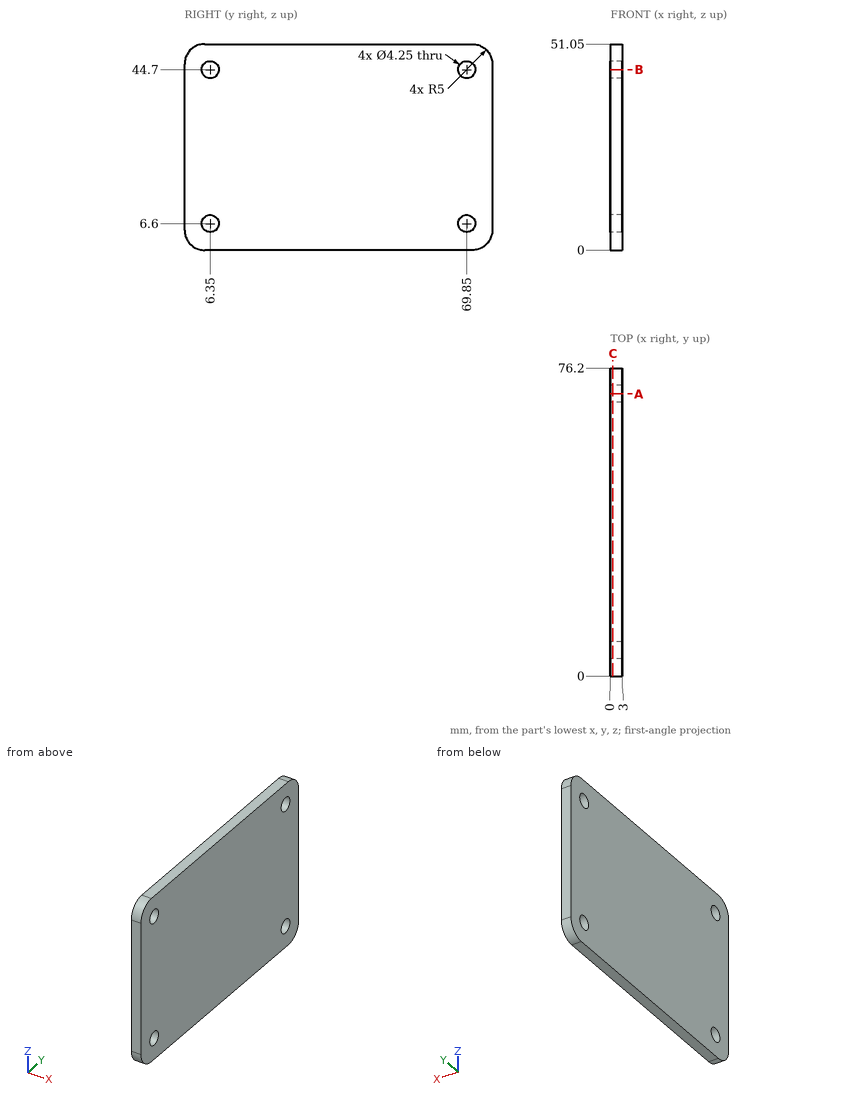
Geometry check sheet. Reference: drawing and pictorial views, mm from the part's lowest x, y, z. Coordinates: 2 decimals unless noted, no trailing zeros. Order: outer loops, then holes, each group sorted by start corner. A loop starts at its lowest first (then second) coordinate and runs counter-clockwise, first axis right, second up.
1. Scan lines: line 1 (Y direction, x = 1.35, z = 44.7) (3 decimals); line 2 (Z direction, x = 1.85, y = 6.35) (3 decimals); line 3 (Y direction, x = 0.7, z = 46). Record each from-to range of solid material in increasing order.
Results found:
line 1: y = 0 to 4.225, 8.475 to 67.725, 71.975 to 76.2
line 2: z = 0 to 4.475, 8.725 to 42.575, 46.825 to 51.05
line 3: y = 0 to 4.67, 8.03 to 68.17, 71.53 to 76.2
2. Sectioned sample at A-A, the plane y = 69.85. Record the cut outline in (x, z) (3 decimals).
Results found:
outline: (0, 0) - (3, 0) - (3, 4.475) - (0, 4.475) - close; (0, 8.725) - (3, 8.725) - (3, 42.575) - (0, 42.575) - close; (0, 46.825) - (3, 46.825) - (3, 51.05) - (0, 51.05) - close
3. Sectioned sample at C-C, the plane x = 0.6. Record the cut outline in (y, z) (3 decimals), and give its area (3 significant figures).
Results found:
outline: (0, 5) arc R5 ccw to (5, 0) - (71.2, 0) arc R5 ccw to (76.2, 5) - (76.2, 46.05) arc R5 ccw to (71.2, 51.05) - (5, 51.05) arc R5 ccw to (0, 46.05) - close; hole circle Ø4.25 at (6.35, 6.6); hole circle Ø4.25 at (6.35, 44.7); hole circle Ø4.25 at (69.85, 6.6); hole circle Ø4.25 at (69.85, 44.7)
area: 3,810 mm2
4. Go/stop test with a flat-tipped pin: pin 1 Ø1.5 at (x, z) = (2, 12.5) entering from -Y. Record where the tip stops, or that it passes through.
Results found:
pin 1: stops at y = 0
5. Sectioned sample at B-B, the plane z = 44.7. Record the cut outline in (x, y) (3 decimals), and give its area (3 significant figures).
Results found:
outline: (0, 0) - (3, 0) - (3, 4.225) - (0, 4.225) - close; (0, 8.475) - (3, 8.475) - (3, 67.725) - (0, 67.725) - close; (0, 71.975) - (3, 71.975) - (3, 76.2) - (0, 76.2) - close
area: 203 mm2
